Verification items for the finished model (mm, model axes). Face numbers are marked on the shaded views. A direction names the side the tool comes from. Give positions to 0.01 mm unless a question says otherwise; leave off trailing zeros. Order: outer loops, then holes, each group sorted by start corner. A loop starts at its lowest first (then second) coordinate and runs counter-clockwise, first axis right, second up. Notation, with made-up numbers: (8, -38.75) -> (55, -38.75) arc R18 ccw to (55, -18.75) -> close; hole circle Ø6 at (4, -15). An arc over 180 degrees is marked (long way). Return JSON: item names as keys, results as strings. Group by question number.
(1) Depth check by flat-ended pin: pin 1 Ø6.5 at (x, z) = (27, 15.5) entering from +Y; pin 2 Ø14.5 at (y, z) = (17, 4.5) entering from -X; pin 3 Ø7 at (y, z) = (-0.5, 3.5) entering from +X; pin 4 Ø5 at (x, y) = (-7.5, -5) entering from +Z. Enter the tip coordinate at first touch or a pass-through.
(2) Cross-section at B-B on y = 17. Enter the section's corners in (x, z).
(3) Cross-section at A-A on x = -24. Enter the section's corners in (y, z), then the cut area to 3 significant figures.
(4) Tool access check on the marked faces 5, 6 and 7. Record the directions out of +Z, -Z, +X, -X, +Y, -Y that give a thin tool (end or side, any length) a straight path to the whole face; none if there is none.
(5) Thickness scan on line 1 along X through (y, z) = (-11, 13.5); line 2 along X through (y, z) = (-2, 9); line 3 along X through (y, z) = (11.5, 6.5). Record the ranges inside material, lowest first.
(6) Cross-section at C-C on y = -14. State how many separate pieces and enclosed holes the cut face has, then the cut area to 3 significant figures.
(7) Cross-section at D-D on x = 0. Enter the section's corners in (y, z).
(8) Release check for a two-part mould opening along X. For the marked faces 1, 2, 3 and 4 record: pulls with the +X half, pulls with the -X half, needs draft (parallel to the pull), parting line crosses it, or undercut.
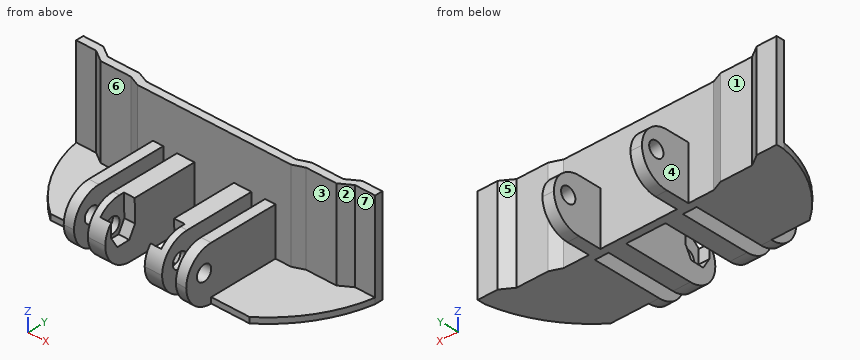
from build123d import *

# Parameters (mm, degrees)
SKETCH2_W                 = 5
SKETCH2_H                 = 25
BOSS_EXTRUDE1_DEPTH       = 14
BOSS_EXTRUDE1_2_DEPTH     = 14
BOSS_EXTRUDE3_DEPTH       = 25
SKETCH5_W                 = 3
SKETCH5_H                 = 13
BOSS_EXTRUDE4_DEPTH       = 14
SKETCH7_W                 = 3
SKETCH7_H                 = 25
BOSS_EXTRUDE5_DEPTH       = 14
SKETCH15_W                = 0.3
SKETCH15_H                = 14
CUT_EXTRUDE2_DEPTH        = 25
SKETCH16_W                = 0.15
SKETCH16_H                = 14
CUT_EXTRUDE3_DEPTH        = 25
FILLET1_R                 = 7
F_4_0MM_DOWEL_HOLE2_D     = 4
FILLET2_R                 = 7
F_4_0MM_DOWEL_HOLE1_D     = 4
F_4_0MM_DOWEL_HOLE1_DEPTH = 26
F_4_0MM_DOWEL_HOLE1_TIP   = 1.201721238
BOSS_EXTRUDE6_DEPTH       = 1.5
CUT_EXTRUDE4_START        = -2.8
SKETCH18_R                = 2
CUT_EXTRUDE4_DEPTH        = 2.8


with BuildPart() as part:
    # Sketch2 → Boss-Extrude1 (new body)
    with BuildSketch(Plane.XY):
        with Locations((-7.5, -6.5)):
            Rectangle(SKETCH2_W, SKETCH2_H)
    extrude(amount=BOSS_EXTRUDE1_DEPTH)



with BuildPart() as body_2:
    # Sketch2 → Boss-Extrude1 2 (new body)
    with BuildSketch(Plane.XY):
        with Locations((7.5, -6.5)):
            Rectangle(SKETCH2_W, SKETCH2_H)
    extrude(amount=BOSS_EXTRUDE1_2_DEPTH)


with BuildPart() as part_1:
    add(part.part)

    add(body_2.part)  # Boss-Extrude3 merges body 2
    # Sketch4 → Boss-Extrude3 (add)
    with BuildSketch(Plane.XY):
        Polygon((-26, 9.206366686), (-30.765993712, 9.206366686), (-33.831204342, 11.206366686), (-39.037863495, 11.206366686), (-39.037863495, 9.206366686), (-33.831204342, 9.206366686), (-30.765993712, 7.206366686), (-26, 7.206366686), align=None)
        Polygon((22.901603942, 7.206366686), (26, 7.206366686), (26, 9.206366686), (22.502408858, 9.206366686), (19.600804916, 8), (10, 8), (-10, 8), (-19.600804916, 8), (-22.502408858, 9.206366686), (-26, 9.206366686), (-26, 7.206366686), (-22.901603942, 7.206366686), (-20, 6), (-10, 6), (10, 6), (20, 6), align=None)
        Polygon((26, 7.206366686), (26, 9.206366686), (30.765993712, 9.206366686), (33.831204342, 11.206366686), (39.037863495, 11.206366686), (39.037863495, 9.206366686), (33.831204342, 9.206366686), (30.765993712, 7.206366686), align=None)
    extrude(amount=BOSS_EXTRUDE3_DEPTH)

    # Sketch5 → Boss-Extrude4 (add)
    with BuildSketch(Plane.XY):
        with Locations((-11.5, 14.5)):
            Rectangle(SKETCH5_W, SKETCH5_H)
        with Locations((11.5, 14.5)):
            Rectangle(SKETCH5_W, SKETCH5_H)
    extrude(amount=BOSS_EXTRUDE4_DEPTH)

    # Sketch7 → Boss-Extrude5 (add)
    with BuildSketch(Plane.XY):
        with Locations((-14.5, -6.5)):
            Rectangle(SKETCH7_W, SKETCH7_H)
        with Locations((14.5, -6.5)):
            Rectangle(SKETCH7_W, SKETCH7_H)
    extrude(amount=BOSS_EXTRUDE5_DEPTH)

    # Sketch15 → Cut-Extrude2 (cut)
    with BuildSketch(Plane.XZ.offset(19)):
        with Locations((-9.85, 7)):
            Rectangle(SKETCH15_W, SKETCH15_H)
        with Locations((9.85, 7)):
            Rectangle(SKETCH15_W, SKETCH15_H)
        with Locations((-13.15, 7)):
            Rectangle(SKETCH15_W, SKETCH15_H)
        with Locations((13.15, 7)):
            Rectangle(SKETCH15_W, SKETCH15_H)
    extrude(amount=-CUT_EXTRUDE2_DEPTH, mode=Mode.SUBTRACT)

    # Sketch16 → Cut-Extrude3 (cut)
    with BuildSketch(Plane.XZ.offset(19)):
        with Locations((-5.075, 7)):
            Rectangle(SKETCH16_W, SKETCH16_H)
        with Locations((5.075, 7)):
            Rectangle(SKETCH16_W, SKETCH16_H)
    extrude(amount=-CUT_EXTRUDE3_DEPTH, mode=Mode.SUBTRACT)

    # Fillet1
    fillet1_edges = [part_1.edges().sort_by_distance(p)[0] for p in [
        (7.425, -19, 14),
        (7.425, -19, 0),
        (-7.425, -19, 0),
        (-7.425, -19, 14),
        (-14.65, -19, 0),
        (-14.65, -19, 14),
        (14.65, -19, 14),
        (14.65, -19, 0),
    ]]
    fillet(fillet1_edges, radius=FILLET1_R - 0.0001)  # a hair under: the kernel refuses the full size

    # Ø4.0mm Dowel Hole2 (through all)
    with Locations(Plane(origin=(16, 0, 0), x_dir=(0, 0, -1), z_dir=(1, 0, 0))):
        with Locations((-8, -14)):
            Hole(F_4_0MM_DOWEL_HOLE2_D / 2)

    # Fillet2
    fillet2_edges = [part_1.edges().sort_by_distance(p)[0] for p in [
        (-11.5, 21, 0),
        (-11.5, 21, 14),
        (11.5, 21, 0),
        (11.5, 21, 14),
    ]]
    fillet(fillet2_edges, radius=FILLET2_R - 0.0001)  # a hair under: the kernel refuses the full size

    # Ø4.0mm Dowel Hole1
    with Locations(Plane(origin=(13, 0, 0), x_dir=(0, 0, -1), z_dir=(1, 0, 0))):
        with Locations((-8, 17)):
            Hole(F_4_0MM_DOWEL_HOLE1_D / 2, depth=F_4_0MM_DOWEL_HOLE1_DEPTH)
            with Locations((0, 0, -(F_4_0MM_DOWEL_HOLE1_DEPTH + F_4_0MM_DOWEL_HOLE1_TIP / 2))):  # 118° drill point
                Cone(0, F_4_0MM_DOWEL_HOLE1_D / 2, F_4_0MM_DOWEL_HOLE1_TIP, mode=Mode.SUBTRACT)

    # Sketch14 → Boss-Extrude6 (add)
    with BuildSketch(Plane.XY):
        with BuildLine():
            Line((-22.901603942, 7.206366686), (-30.765993712, 7.206366686))
            Line((-30.765993712, 7.206366686), (-33.831204342, 9.206366686))
            Line((-33.831204342, 9.206366686), (-39.037863495, 9.206366686))
            ThreePointArc((-39.037863495, 9.206366686), (-34.518223809, -2.625999259), (-26, -12))
            Line((-26, -12), (-16, -12))
            Line((-16, -12), (-16, 6))
            Line((-16, 6), (-20, 6))
            Line((-20, 6), (-22.901603942, 7.206366686))
        make_face()
        with BuildLine():
            Line((20, 6), (16, 6))
            Line((16, 6), (16, -12))
            Line((16, -12), (26, -12))
            ThreePointArc((26, -12), (34.518223809, -2.625999259), (39.037863495, 9.206366686))
            Line((39.037863495, 9.206366686), (33.831204342, 9.206366686))
            Line((33.831204342, 9.206366686), (30.765993712, 7.206366686))
            Line((30.765993712, 7.206366686), (22.901603942, 7.206366686))
            Line((22.901603942, 7.206366686), (20, 6))
        make_face()
    extrude(amount=BOSS_EXTRUDE6_DEPTH)

    # Sketch18 → Cut-Extrude4 (cut)
    # profile 1 of 3: a face of its own
    with BuildSketch(Plane(origin=(-5.15, 0, 0), x_dir=(0, 0, -1), z_dir=(1, 0, 0)).offset(CUT_EXTRUDE4_START)):
        Polygon((-7.940827202, -17.348108707), (-5.070866406, -15.622809207), (-5.130039204, -12.2747005), (-8.059172798, -10.651891293), (-10.929133594, -12.377190793), (-10.869960796, -15.7252995), align=None)
        with Locations((-8, -14)):
            Circle(SKETCH18_R, mode=Mode.SUBTRACT)
    # profile 2 of 3: a face of its own
    with BuildSketch(Plane(origin=(-5.15, 0, 0), x_dir=(0, 0, -1), z_dir=(1, 0, 0)).offset(CUT_EXTRUDE4_START)):
        with BuildLine():
            Line((-22.212279743, -17.348108707), (-11.516384977, -17.348108707))
            ThreePointArc((-11.516384977, -17.348108707), (-13.348806771, -14.948330474), (-14, -12))
            Line((-14, -12), (-14, -10.7568865))
            Line((-14, -10.7568865), (-22.212279743, -10.902026223))
            Line((-22.212279743, -10.902026223), (-22.212279743, -17.348108707))
        make_face()
    # profile 3 of 3: a face of its own
    with BuildSketch(Plane(origin=(-5.15, 0, 0), x_dir=(0, 0, -1), z_dir=(1, 0, 0)).offset(CUT_EXTRUDE4_START)):
        with BuildLine():
            Line((-11.516384977, -17.348108707), (-7.940827202, -17.348108707))
            Line((-7.940827202, -17.348108707), (-10.869960796, -15.7252995))
            Line((-10.869960796, -15.7252995), (-10.929133594, -12.377190793))
            Line((-10.929133594, -12.377190793), (-8.059172798, -10.651891293))
            Line((-8.059172798, -10.651891293), (-14, -10.7568865))
            Line((-14, -10.7568865), (-14, -12))
            ThreePointArc((-14, -12), (-13.348806771, -14.948330474), (-11.516384977, -17.348108707))
        make_face()
    cut_extrude4 = extrude(amount=CUT_EXTRUDE4_DEPTH, mode=Mode.SUBTRACT)

    # Mirror1: Cut-Extrude4 across plane
    add(cut_extrude4.mirror(Plane(origin=(0, 0, 0), x_dir=(0, 0, 1), z_dir=(1, 0, 0))), mode=Mode.SUBTRACT)


solid = part_1.part
Verdict:
{
 "1": {"pin 1": "y = 9.21", "pin 2": "x = -39.04", "pin 3": "x = 37.05", "pin 4": "z = 14"},
 "2": {"outline": "(-13, 0.68) -> (-10, 0.68) -> (-10, 6) -> (-13, 6) -> close; (-13, 10) -> (-10, 10) -> (-10, 13.32) -> (-13, 13.32) -> close; (10, 0.68) -> (13, 0.68) -> (13, 6) -> (10, 6) -> close; (10, 10) -> (13, 10) -> (13, 13.32) -> (10, 13.32) -> close"},
 "3": {"outline": "(-12, 0) -> (9.21, 0) -> (9.21, 25) -> (7.21, 25) -> (7.21, 1.5) -> (-12, 1.5) -> close", "area": "78.8 mm²"},
 "4": {"face 5": "+Z, -Z, +Y", "face 6": "+Z, -X, -Y", "face 7": "+Z, +X, -Y"},
 "5": {"line 1": "-16 to -13.3, -9.7 to -7.95, 7.95 to 9.7, 13.3 to 16", "line 2": "-16 to -13.3, -9.7 to -5.15, 5.15 to 9.7, 13.3 to 16", "line 3": "-13 to -10, 10 to 13"},
 "6": {"separate pieces": "8", "enclosed holes": "0", "area": "111 mm²"},
 "7": {"outline": "(6, 0) -> (8, 0) -> (8, 25) -> (6, 25) -> close"},
 "8": {"face 1": "undercut", "face 2": "pulls with the +X half", "face 3": "needs draft", "face 4": "undercut"}
}
